Part print with two shaded views. Sizes in mm from the minimum x, y, z corner. A direction names the side the tool comes from. Give positions to 0.01 mm unless a question says otherwise; leave off trailing zeros. Write each loop counter-clockwise with the first axis right and the second up, starting at its lowest first coordinate (ties: lowest second). Pieces come first, ordered by that corner, then holes.
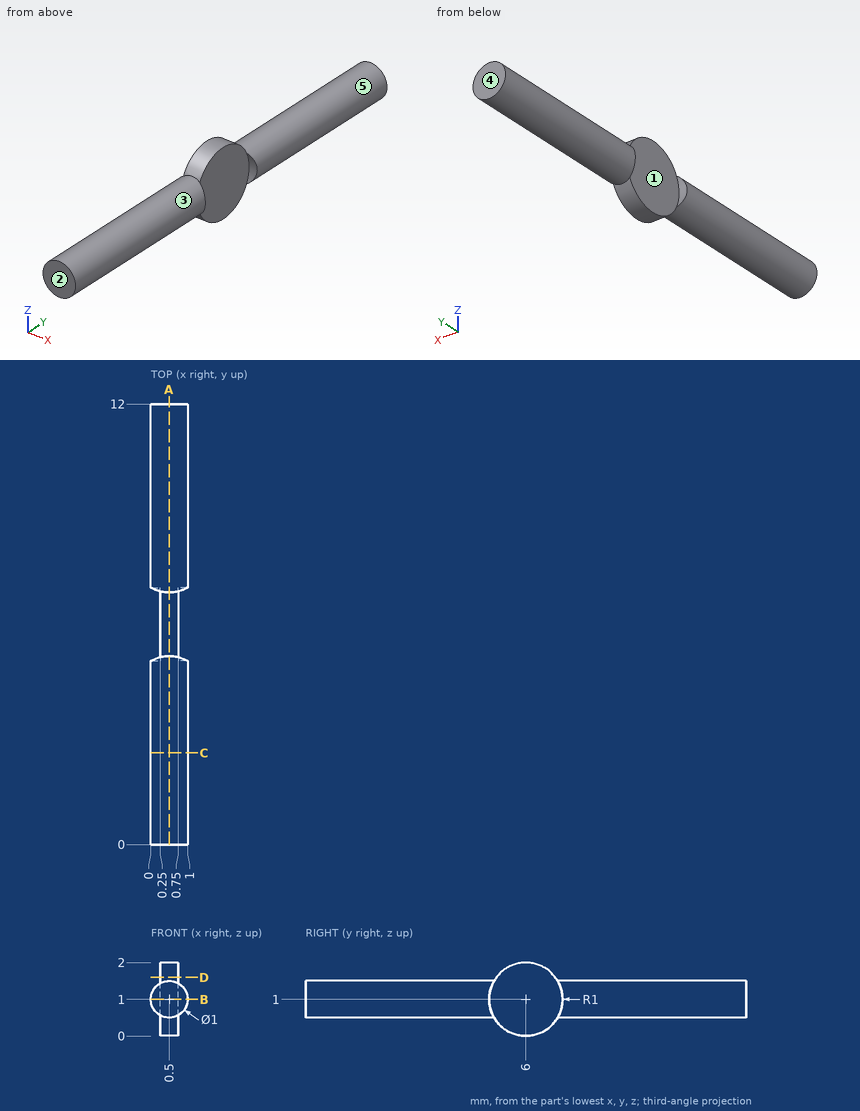
1) Saw through at B-B, the plane z = 1. Write the cut outline in (x, y), then the cut area to 3 significant figures.
Answers follow:
outline: (0, 0) - (1, 0) - (1, 5) - (0.75, 5) - (0.75, 7) - (1, 7) - (1, 12) - (0, 12) - (0, 7) - (0.25, 7) - (0.25, 5) - (0, 5) - close
area: 11.0 mm2
2) 3-axis set-ups, long thin cutter, end or side, ignore diameter. For the marked faces 4 and 5: which of +Z, -Z, +X, -X, +Y, -Y reach the whole face in a straight line?
Answers follow:
face 4: +Z, -Z, +X, -X, +Y
face 5: +Y
3) Wall check: L1, parallel to Y at x = 0.85, z = 0.75; L2, parallel to Y at x = 0.7, z = 0.45; L3, parallel to X at y = 10.75, z = 0.85. Give the ranges that are in metal, low to high.
Answers follow:
L1: y = 0 to 5.03, 6.97 to 12
L2: y = 5.16 to 6.84
L3: x = 0.02 to 0.98
4) Saw through at A-A, the plane x = 0.5. Write the cut outline in (y, z), then the cut area to 3 significant figures.
Answers follow:
outline: (0, 0.5) - (5.13, 0.5) arc R1 ccw to (6.87, 0.5) - (12, 0.5) - (12, 1.5) - (6.87, 1.5) arc R1 ccw to (5.13, 1.5) - (0, 1.5) - close
area: 13.2 mm2
5) Saw through at D-D, the plane z = 1.6. Write the cut outline in (x, y).
Answers follow:
outline: (0.25, 5.2) - (0.75, 5.2) - (0.75, 6.8) - (0.25, 6.8) - close
6) Two-plate mould, pull along Y, no slides. Class the marked faces 1, 2 and 3: +Y half, -Y half, draft (parallel to the pull), parting line (faces both ways), or undercut.
Answers follow:
face 1: undercut
face 2: -Y half
face 3: draft
7) Saw through at C-C, the plane y = 2.5. Write the cut outline in (x, z), then the cut area to 3 significant figures.
Answers follow:
outline: circle Ø1 at (0.5, 1)
area: 0.785 mm2
